Autodesk Inventor part; units mm, degrees
ref_plane "YZ Plane" through (0, 0, 0) normal (1, 0, 0) x (0, 1, 0)
ref_plane "XZ Plane" through (0, 0, 0) normal (0, 1, 0) x (-1, 0, 0)
ref_plane "XY Plane" through (0, 0, 0) normal (0, 0, 1) x (1, 0, 0)
sketch "Sketch1" plane through (0, 0, 0) normal (0, 0, 1) x (1, 0, 0)
  line L0 (0, 0) -> (25.4, 0)
  line L1 (25.4, 0) -> (25.4, 25.4)
  line L2 (25.4, 25.4) -> (0, 25.4)
  line L3 (0, 25.4) -> (0, 0)
  dimension "d0" = 25.4
  dimension "d1" = 25.4
extrude "Extrusion1" add sketch "Sketch1" along normal blind 381
shell "Shell1" thickness 1.5875 removed faces 2 at (16.9333, 16.9333, 0) at (16.9333, 16.9333, 381)
sketch "Sketch2" plane through (25.4, 0, 0) normal (1, 0, 0) x (0, 0, -1)
  line L0 (-381, 25.4) -> (-381, 0)
  line L1 (0, 0) -> (0, 25.4)
  line L2 (0, 25.4) -> (-381, 25.4)
  line L3 (-381, 0) -> (-355.6, 25.4)
  line L4 (-381, 25.4) -> (-381, 0)
  line L5 (-381, 25.4) -> (-355.6, 25.4)
  line L6 (0, 25.4) -> (-25.4, 25.4)
  line L7 (0, 0) -> (-25.4, 25.4)
  line L8 (0, 0) -> (0, 25.4)
  dimension "d6" = 45
  dimension "d7" = 45
extrude "Extrusion2" cut sketch "Sketch2" against normal through all
sketch "Sketch3" plane through (0, 25.4, 355.6) normal (0, 1, 0) x (1, 0, 0)
  line L0 (25.4, 330.2) -> (25.4, 0)
  line L1 (25.4, 330.2) -> (0, 330.2)
  circle A0 centre (12.7, 190.5) radius 3.175
  point P0 (0, 355.6)
  dimension "d10" = 6.35
  dimension "d11" = 12.7
  dimension "d12" = 139.7
extrude "Extrusion3" cut sketch "Sketch3" against normal through all
properties part number "Frame_RearLowerAngleSupport"
Source: CAD feature listing. Evaluate the final solid. Frame: model axes, mm. A direction names the side the tool comes from. Coordinates: 2 decimals unless noted, no trailing zeros. Loops run counter-clockwise (first coordinate to the right, second up) from the corner with the lowest first, then second, coordinate; pieces in that order, holes last. Notation, with made-up numbers: (-18, 20.25) -> (40, 20.25) arc R23 cw to (40, 35.25) -> close; hole circle Ø6 at (25.25, 38.25). An arc over 180 degrees is marked (long way). One line per item, written item: value. Start each with the question number.
Q1. Section query A-A, the plane z = 165.1. Return the cut outline in (x, y) (1 decimal), and give its area (3 significant figures).
Q2. Section query B-B, the plane y = 6.5. Return the cut outline in (x, z).
Q3. Section query C-C, the plane x = 12.7. Return the cut outline in (y, z) (1 decimal), and give its area (3 significant figures).
Q4. Section query D-D, the plane z = 76.5. Return the cut outline in (x, y).
Q5. Line query: line 1 along X through (y, z) = (1.75, 125); line 2 along X through (y, z) = (25.15, 165.1) (3 decimals). Output: solid intervals per line, ascending.
Q6. Mould query, pull axis X, two halves, no side actions, for faces 1 (the face through (23.812, 13, 188)), 2 (the face through (13, 0, 188)), 3 (the face through (25.4, 13, 188)). Classes: pulls with the +X half, pulls with the -X half, needs draft (parallel to the pull), parting line crosses it, or undercut.
Q7. Set-up query: faces 4 (the face through (1.588, 13, 188)), 5 (the face through (24, 13, 13)). Return all of +Z, -Z, +X, -X, +Y, -Y with unobstructed straight access to the full face (end or side cutting, diameter ignored); none if empty.
Results:
1. outline: (0, 0) -> (9.5, 0) -> (9.5, 1.6) -> (1.6, 1.6) -> (1.6, 23.8) -> (9.5, 23.8) -> (9.5, 25.4) -> (0, 25.4) -> close; (15.9, 0) -> (25.4, 0) -> (25.4, 25.4) -> (15.9, 25.4) -> (15.9, 23.8) -> (23.8, 23.8) -> (23.8, 1.6) -> (15.9, 1.6) -> close
1. area: 131 mm^2
2. outline: (0, 6.5) -> (1.59, 6.5) -> (1.59, 374.5) -> (0, 374.5) -> close; (23.81, 6.5) -> (25.4, 6.5) -> (25.4, 374.5) -> (23.81, 374.5) -> close
3. outline: (0, 0) -> (1.6, 1.6) -> (1.6, 161.9) -> (0, 161.9) -> close; (0, 168.3) -> (1.6, 168.3) -> (1.6, 379.4) -> (0, 381) -> close; (23.8, 23.8) -> (25.4, 25.4) -> (25.4, 161.9) -> (23.8, 161.9) -> close; (23.8, 168.3) -> (25.4, 168.3) -> (25.4, 355.6) -> (23.8, 357.2) -> close
3. area: 1,110 mm^2
4. outline: (0, 0) -> (25.4, 0) -> (25.4, 25.4) -> (0, 25.4) -> close; hole (1.59, 1.59) -> (23.81, 1.59) -> (23.81, 23.81) -> (1.59, 23.81) -> close
5. line 1: 0 to 1.59, 23.81 to 25.4
5. line 2: 0 to 9.525, 15.875 to 25.4
6. face 1: undercut
6. face 2: needs draft
6. face 3: pulls with the +X half
7. face 4: +Z, -Z
7. face 5: -Z, +X, -X, +Y
